Could you check a few things on this model? Use its own coordinates, in mm. A direction names the side the tool comes from. Give positions to 0.01 mm unless a question says otherwise; leave off trailing zeros. Order: outer loops, then holes, each group sorted by start corner. A loop starts at its lowest first (then second) coordinate and runs counter-clockwise, first axis right, second up.
(1) Will these pins go through, and if not, where does the flat tip stop? pin 1 (6 mm diameter, centred on y = 7, z = 43, fed in from +X); pin 2 (5 mm diameter, centred on y = 12.5, z = 27, fed in from -X); pin 3 (12 mm diameter, centred on y = 6, z = 36.5, fed in from -X); pin 4 (4.5 mm diameter, centred on x = 0, z = 0, fed in from +Y).
(2) On a 3-axis mill with a long thin cutter (end or side, diameter ignored), from which of +Z, -Z, +X, -X, +Y, -Y can I reach the whole of each face in a straight line? I mean faces 1 (the cylindrical face through (-28.17, 10.81, 58.99)), 2 (the flat face through (0, 10, 60)), 3 (the flat face through (23, 8, 58)). Say none if no direction works.
(3) Imagine slicing it at A-A, the plane x = 0. Write out the boundary of the cut face in (y, z), then the cut area to 3 significant figures.
(4) Imagine slicing it at C-C, the plane z = 43. Write out the boundary of the cut face in (x, y).
(5) If I drill on probe 1 along X at (y, z) = (17.75, 55); probe 2 along X at (y, z) = (16, 22.5); probe 3 along X at (y, z) = (11.25, 30), over which ranges is the centre line in solid material (lowest first)?
(6) Imagine slicing it at B-B, the plane y = 14. State how many separate pieces and enclosed holes the cut face has, then the cut area to 3 significant figures.
(7) If we mould it in two halves opening along X, with no side actions, what happens to faces 4 (the flat face through (-16.8, 10, 45)), 5 (the flat face through (0, 20, 37)), 6 (the flat face through (20.26, 9.86, 25.41))? For each: released by +X, released by -X, zero draft, split by the parting line, or undercut.
(8) Imagine slicing it at D-D, the plane x = 25. Write out the boundary of the cut face in (y, z), then the cut area to 3 significant figures.
from build123d import *

# Parameters (mm, degrees)
SALIENTE_EXTRUIR1_DEPTH = 20
CORTAR_EXTRUIR1_START   = -20
CORTAR_EXTRUIR1_DEPTH   = 20
CROQUIS3_R              = 2.6
CORTAR_EXTRUIR2_DEPTH   = 20
CROQUIS4_R              = 2.7
CORTAR_EXTRUIR3_DEPTH   = 20


with BuildPart() as part:
    # Croquis1 → Saliente-Extruir1 (new body)
    with BuildSketch(Plane(origin=(0, 0, 0), x_dir=(1, 0, 0), z_dir=(0, 1, 0))):
        with BuildLine():
            Line((-4.342546511, 2.47836434), (-35.731971676, -52.52163566))
            ThreePointArc((-35.731971676, -52.52163566), (-35.713301997, -57.510794525), (-31.389425165, -60))
            Line((-31.389425165, -60), (31.389425165, -60))
            ThreePointArc((31.389425165, -60), (35.713301997, -57.510794525), (35.731971676, -52.52163566))
            Line((35.731971676, -52.52163566), (4.342546511, 2.47836434))
            ThreePointArc((4.342546511, 2.47836434), (0, 5), (-4.342546511, 2.47836434))
        make_face()
    extrude(amount=SALIENTE_EXTRUIR1_DEPTH)

    # Croquis2 → Cortar-Extruir1 (cut)
    with BuildSketch(Plane(origin=(0, 20, 0), x_dir=(1, 0, 0), z_dir=(0, 1, 0)).offset(CORTAR_EXTRUIR1_START)):
        with BuildLine():
            Line((-19.800240489, -58), (-19.800240489, -28.641255076))
            Line((-19.800240489, -28.641255076), (-33.994953072, -53.512981396))
            ThreePointArc((-33.994953072, -53.512981396), (-33.983751264, -56.506476715), (-31.389425165, -58))
            Line((-31.389425165, -58), (-19.800240489, -58))
        make_face()
        Polygon((-16.800240489, -58), (-3.194307375, -58), (-16.800240489, -32.094821088), align=None)
        with BuildLine():
            Line((-1.5, -54.77410323), (-1.5, -4.769696007))
            ThreePointArc((-1.5, -4.769696007), (-3.347002716, -3.714508422), (-4.588219379, -1.987018604))
            Line((-4.588219379, -1.987018604), (-17.417918454, -24.466992207))
            Line((-17.417918454, -24.466992207), (-1.5, -54.77410323))
        make_face()
        with BuildLine():
            ThreePointArc((4.588219379, -1.987018604), (3.347002716, -3.714508422), (1.5, -4.769696007))
            Line((1.5, -4.769696007), (1.5, -54.77410323))
            Line((1.5, -54.77410323), (17.417918454, -24.466992207))
            Line((17.417918454, -24.466992207), (4.588219379, -1.987018604))
        make_face()
        with BuildLine():
            Line((33.994953072, -53.512981396), (19.800240489, -28.641255076))
            Line((19.800240489, -28.641255076), (19.800240489, -58))
            Line((19.800240489, -58), (31.389425165, -58))
            ThreePointArc((31.389425165, -58), (33.983751264, -56.506476715), (33.994953072, -53.512981396))
        make_face()
        Polygon((16.800240489, -32.094821088), (3.194307375, -58), (16.800240489, -58), align=None)
    extrude(amount=CORTAR_EXTRUIR1_DEPTH, mode=Mode.SUBTRACT)

    # Croquis3 → Cortar-Extruir2 (cut)
    with BuildSketch(Plane(origin=(0, 20, 0), x_dir=(1, 0, 0), z_dir=(0, 1, 0))):
        with Locations(Location((0, 0, 0), (0, 0, 270))):
            Circle(CROQUIS3_R)
    extrude(amount=-CORTAR_EXTRUIR2_DEPTH, mode=Mode.SUBTRACT)

    # Croquis4 → Cortar-Extruir3 (cut)
    with BuildSketch(Plane(origin=(0, 0, 58), x_dir=(-1, 0, 0), z_dir=(0, 0, -1))):
        with Locations((25.594832827, 10)):
            Circle(CROQUIS4_R)
        with Locations((-25.594832827, 10)):
            Circle(CROQUIS4_R)
    extrude(amount=-CORTAR_EXTRUIR3_DEPTH, mode=Mode.SUBTRACT)


solid = part.part
Answer block:
1. pin 1: stops at x = 32.01
1. pin 2: stops at x = -22.59
1. pin 3: stops at x = -30.01
1. pin 4: passes through
2. face 1: +Z
2. face 2: +Z, +X, -X, +Y, -Y
2. face 3: +Y, -Y
3. outline: (0, -5) - (20, -5) - (20, -2.6) - (0, -2.6) - close; (0, 2.6) - (20, 2.6) - (20, 60) - (0, 60) - close
3. area: 1,200 mm2
4. outline: (-30.3, 0) - (-28, 0) - (-28, 20) - (-30.3, 20) - close; (-19.8, 0) - (-16.8, 0) - (-16.8, 20) - (-19.8, 20) - close; (-11.07, 0) - (-7.68, 0) - (-7.68, 20) - (-11.07, 20) - close; (-1.5, 0) - (1.5, 0) - (1.5, 20) - (-1.5, 20) - close; (7.68, 0) - (11.07, 0) - (11.07, 20) - (7.68, 20) - close; (16.8, 0) - (19.8, 0) - (19.8, 20) - (16.8, 20) - close; (28, 0) - (30.3, 0) - (30.3, 20) - (28, 20) - close
5. probe 1: x = -36.39 to -34.39, -19.8 to -16.8, -4.77 to 4.77, 16.8 to 19.8, 34.39 to 36.39
5. probe 2: x = -18.6 to -16.3, -1.5 to 1.5, 16.3 to 18.6
5. probe 3: x = -22.88 to -20.58, -19.8 to -14.51, -1.5 to 1.5, 14.51 to 19.8, 20.58 to 22.88
6. separate pieces: 1
6. enclosed holes: 7
6. area: 1,000 mm2
7. face 4: undercut
7. face 5: zero draft
7. face 6: released by +X
8. outline: (0, 33.72) - (20, 33.72) - (20, 37.75) - (0, 37.75) - close; (0, 58) - (7.37, 58) - (7.37, 60) - (0, 60) - close; (12.63, 58) - (20, 58) - (20, 60) - (12.63, 60) - close
8. area: 110 mm2
